Build history of the part. All positions in model axes, mm. Face numbers are marked on the shaded views. A direction names the side the tool comes from. Give positions to 0.01 mm unless a question says otherwise; leave off trailing zeros. Order: outer loops, then holes, each group sorted by start corner. A loop starts at its lowest first (then second) coordinate and runs counter-clockwise, first axis right, second up. Notation, with made-up numbers: M 32.25,71 L 79.25,71 A25 cw 79.25,94 Z; hole C -1,23.5 d11. An arc over 180 degrees is marked long. Answer as CSV lines item,"result".
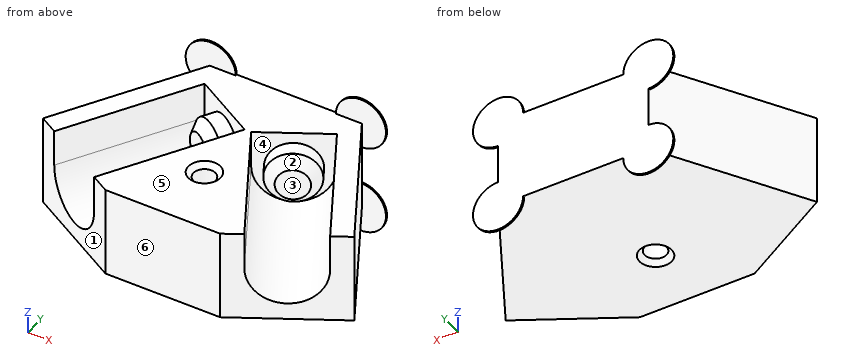
from build123d import *

# Parameters (mm, degrees)
F0_R      = 3.25
F1_DEPTH  = 31.5
F3_DEPTH  = 43
F5_DEPTH  = 43
F6_R      = 7.625
F7_DEPTH  = 7.5
F8_R      = 7.625
F9_DEPTH  = 7.5
F10_SIZE  = 3
F11_DEPTH = 5
F12_SIZE  = 1.5
F13_R     = 7.5
F14_DEPTH = 0.5


with BuildPart() as f1:
    # F0 (on Top) → F1 (new body)
    with BuildSketch(Plane.XY):
        Polygon((22.5, 195.0052188787), (-22.5, 195.0052188787), (-46.6147367097, 153.2372696863), (-17.1698729811, 136.2372696863), (17.1698729811, 136.2372696863), (46.6147367097, 153.2372696863), align=None)
        with Locations((0, 155.976362049)):
            Circle(F0_R, mode=Mode.SUBTRACT)
    extrude(amount=F1_DEPTH)

    # F2 (on face) → F3 (cut)
    with BuildSketch(Plane(origin=(54.7, 94.743179174, 0), x_dir=(0.8660254038, -0.5, 0), z_dir=(-0.5, -0.8660254038, 0))):
        with BuildLine():
            Line((-110.8631810245, 31.5), (-110.8631810245, 15.75))
            ThreePointArc((-110.8631810245, 15.75), (-99.9881810245, 4.875), (-89.1131810245, 15.75))
            Line((-89.1131810245, 15.75), (-89.1131810245, 31.5))
            Line((-89.1131810245, 31.5), (-110.8631810245, 31.5))
        make_face()
    extrude(amount=-F3_DEPTH, mode=Mode.SUBTRACT)

    # F4 (on face) → F5 (cut)
    with BuildSketch(Plane(origin=(-54.7, 94.743179174, 0), x_dir=(0.8660254038, 0.5, 0), z_dir=(0.5, -0.8660254038, 0))):
        with BuildLine():
            Line((89.1131810245, 31.5), (89.1131810245, 15.75))
            ThreePointArc((89.1131810245, 15.75), (99.9881810245, 4.875), (110.8631810245, 15.75))
            Line((110.8631810245, 15.75), (110.8631810245, 31.5))
            Line((110.8631810245, 31.5), (89.1131810245, 31.5))
        make_face()
    extrude(amount=-F5_DEPTH, mode=Mode.SUBTRACT)

    # F6 (on face) → F7 (join)
    with BuildSketch(Plane(origin=(76.2, 131.9822715367, 0), x_dir=(0.8660254038, -0.5, 0), z_dir=(-0.5, -0.8660254038, 0))):
        with Locations((-99.9881810245, 15.75)):
            Circle(F6_R)
    extrude(amount=F7_DEPTH)

    # F8 (on face) → F9 (join)
    with BuildSketch(Plane(origin=(-76.2, 131.9822715367, 0), x_dir=(0.8660254038, 0.5, 0), z_dir=(0.5, -0.8660254038, 0))):
        with Locations((99.9881810245, 15.75)):
            Circle(F8_R)
    extrude(amount=F9_DEPTH)

    # F10
    f10_edges = [f1.edges().sort_by_distance(p)[0] for p in [
        (-20.745749, 179.293672, 15.75),
        (7.538861, 171.668672, 15.75),
    ]]
    chamfer(f10_edges, length=F10_SIZE)

    # F11 (cut): a face of the model
    f11_faces = [f1.faces().sort_by_distance(p)[0] for p in [
        (0, 166.034633576, 31.5),
    ]]
    extrude(f11_faces, amount=-F11_DEPTH, mode=Mode.SUBTRACT)

    # F12
    f12_edges = [f1.edges().sort_by_distance(p)[0] for p in [
        (-3.25, 155.976362, 26.5),
        (-3.25, 155.976362, 0),
    ]]
    chamfer(f12_edges, length=F12_SIZE)

    # F13 (on face) → F14 (join)
    with BuildSketch(Plane(origin=(0, 195.0052188787, 0), x_dir=(-1, 0, 0), z_dir=(0, 1, 0))):
        with Locations((-22.5, 26.5)):
            Circle(F13_R)
        with Locations((22.5, 26.5)):
            Circle(F13_R)
        with Locations((22.5, 0)):
            Circle(F13_R)
        with Locations((-22.5, 0)):
            Circle(F13_R)
    extrude(amount=-F14_DEPTH)


solid = f1.part
Item 1: Drop flat-ended pins along their axis: pin 1 (2 mm diameter, centred on y = 148.5, z = 12.5, fed in from -X); pin 2 (1.5 mm diameter, centred on x = -30, y = 169.5, fed in from +Z); pin 3 (8 mm diameter, centred on x = -37, z = 6.5, fed in from +Y). Give the stop position or say it passes through.
Geometry says:
pin 1,"stops at x = -18.44"
pin 2,"stops at z = 26.5"
pin 3,"stops at y = 176.82"
Item 2: Pull direction Z, two halves, no side cores. Call the marked faces 4, 5 and 6: released by +Z, released by -Z, zero draft, split by the parting line, or undercut.
Geometry says:
face 4,"undercut"
face 5,"released by +Z"
face 6,"zero draft"
Item 3: Band-saw the part on A-A (x = 0). Give the cut face in (y, z).
Geometry says:
outline,"M 136.24,0 L 151.23,0 L 152.73,1.5 L 152.73,25 L 151.23,26.5 L 136.24,26.5 Z; M 159.23,1.5 L 160.73,0 L 195.01,0 L 195.01,26.5 L 160.73,26.5 L 159.23,25 Z"
Item 4: 3-axis set-ups, long thin cutter, end or side, ignore diameter. For the marked faces 1, 2 and 3: which of +Z, -Z, +X, -X, +Y, -Y reach the whole face in a straight line?
Geometry says:
face 1,"+Z, -Z, -X, -Y"
face 2,"none"
face 3,"+Z"
Item 5: Probe line 1 along Y through (x, z) = (0, 15); line 2 along X through (y, z) = (170, 8.5); line 3 along X through (y, z) = (167, 13). List the from-to ranges inside material, lowest first. Write a range as from..to.
Geometry says:
line 1,"y = 136.24..152.73, 159.23..195.01"
line 2,"x = -36.94..-26.67, -7.95..7.95, 26.67..36.94"
line 3,"x = -38.67..-31.19, -6.89..6.89, 31.19..38.67"
Item 6: Band-saw the part on B-B (x = 25). State how many separate pieces and enclosed holes the cut face has, and give its area (3 significant figures).
Geometry says:
separate pieces,"3"
enclosed holes,"0"
area,"590 mm2"
